Part model, mm, in its own coordinate system. A direction names the side the tool comes from. Coordinates: 2 decimals unless noted, no trailing zeros. Write each loop counter-clockwise with the first axis right and the second up, starting at its lowest first coordinate (ties: lowest second). Pieces come first, ordered by that corner, then holes. Notation, with made-up numbers: (85, 49.25) -> (126, 49.25) arc R29 cw to (126, 82.25) -> close; hole circle Ø8 at (65, 9). An arc over 180 degrees is marked (long way). Write item = value, one per line. Start each with the question number.
Q1. Band-saw the part on B-B, the plane z = 143. List the corners of the cut face in (x, y), plus the area to 3 significant figures.
Q2. Pull direction Y, two halves, no side cores. Call faces 1 (the cylindrical face through (5.8, -0.49, 141.06)), 2 (the cylindrical face through (9.51, -2.9, 27.09)), 3 (the flat face through (5, 0, 73)): released by +Y, released by -Y, zero draft, split by the parting line, or undercut.
Q3. Pin check, flat tip, straight feed: P1, Ø1, axis at x = 2, y = -4.5, coming from the -Z side. Stop position of the tip, or through.
Q4. Probe line 1 (X direction, y = -2.75, z = 62.5); line 2 (Y direction, x = 3.5, z = 106); line 3 (Y direction, x = 9.5, z = 27). List the from-to ranges inside material, lowest first.
Q5. Band-saw the part on C-C, the plane z = 10. List the corners of the cut face in (x, y), plus the area to 3 significant figures.
Q6. Band-saw the part on D-D, the plane y = -4.5. List the corners of the cut face in (x, z).
Q7. Tool access for faces 4 (the cylindrical face through (5.09, -9.49, 34.9)), 5 (the flat face through (5, -9, 73)): list every direction of +Z, -Z, +X, -X, +Y, -Y with a clear straight run to the whole face (end or side of a thin tool).
Q8. Band-saw the part on A-A, the plane x = 5. Give the number of separate pieces and of enclosed holes in the cut face, plus the area to 3 significant figures.
from build123d import *

# Parameters (mm, degrees)
SKETCH_1_W               = 10
SKETCH_1_H               = 10
SKETCH_1_W_2             = 8
SKETCH_1_H_2             = 8
EXTRUDE_1_DEPTH          = 148
CUT_EXTRUDE_1_DEPTH      = 149.67414032
CUT_EXTRUDE_1_DEPTH_BACK = 149.67414032
SKETCH_2_R               = 2.1
SKETCH_3_R               = 2.1
CUT_EXTRUDE_2_DEPTH      = 149.67414032


with BuildPart() as part:
    # 草图1 → 拉伸-薄壁1 (new body)
    with BuildSketch(Plane.XY):
        with Locations((5, -5)):
            Rectangle(SKETCH_1_W, SKETCH_1_H)
        with Locations((5, -5)):
            Rectangle(SKETCH_1_W_2, SKETCH_1_H_2, mode=Mode.SUBTRACT)
    extrude(amount=EXTRUDE_1_DEPTH)

    # 草图2 → 切除-拉伸1 (cut, two sides: drawn at the far end of the back side and taken through both)
    with BuildSketch(Plane.ZY.offset(-CUT_EXTRUDE_1_DEPTH_BACK)):
        with Locations(Location((27, -5, 0), (0, 0, 270))):
            Circle(SKETCH_2_R)
        with Locations(Location((47, -5, 0), (0, 0, 270))):
            Circle(SKETCH_2_R)
    extrude(amount=CUT_EXTRUDE_1_DEPTH + CUT_EXTRUDE_1_DEPTH_BACK, mode=Mode.SUBTRACT)

    # 草图3 → 切除-拉伸2 (cut, through all)
    with BuildSketch(Plane(origin=(0, 0, 0), x_dir=(1, 0, 0), z_dir=(0, 1, 0))):
        with Locations(Location((5, -5, 0), (0, 0, 270))):
            Circle(SKETCH_3_R)
        with Locations(Location((5, -143, 0), (0, 0, 90))):
            Circle(SKETCH_3_R)
        with Locations(Location((5, -37, 0), (0, 0, 270))):
            Circle(SKETCH_3_R)
    extrude(amount=-CUT_EXTRUDE_2_DEPTH, mode=Mode.SUBTRACT)


solid = part.part
Ans:
q1.outline = (0, -10) -> (2.9, -10) -> (2.9, -9) -> (1, -9) -> (1, -1) -> (2.9, -1) -> (2.9, 0) -> (0, 0) -> close; (7.1, -10) -> (10, -10) -> (10, 0) -> (7.1, 0) -> (7.1, -1) -> (9, -1) -> (9, -9) -> (7.1, -9) -> close
q1.area = 27.6 mm2
q2.face_1 = zero draft
q2.face_2 = undercut
q2.face_3 = released by +Y
q3.P1 = through
q4.line_1 = 0 to 1, 9 to 10
q4.line_2 = -10 to -9, -1 to 0
q4.line_3 = -10 to -7.1, -2.9 to 0
q5.outline = (0, -10) -> (10, -10) -> (10, 0) -> (0, 0) -> close; hole (1, -9) -> (9, -9) -> (9, -1) -> (1, -1) -> close
q5.area = 36.0 mm2
q6.outline = (0, 0) -> (1, 0) -> (1, 24.96) -> (0, 24.96) -> close; (0, 29.04) -> (1, 29.04) -> (1, 44.96) -> (0, 44.96) -> close; (0, 49.04) -> (1, 49.04) -> (1, 148) -> (0, 148) -> close; (9, 0) -> (10, 0) -> (10, 24.96) -> (9, 24.96) -> close; (9, 29.04) -> (10, 29.04) -> (10, 44.96) -> (9, 44.96) -> close; (9, 49.04) -> (10, 49.04) -> (10, 148) -> (9, 148) -> close
q7.face_4 = +Y, -Y
q7.face_5 = +Z, -Z
q8.separate_pieces = 8
q8.enclosed_holes = 0
q8.area = 271 mm2
